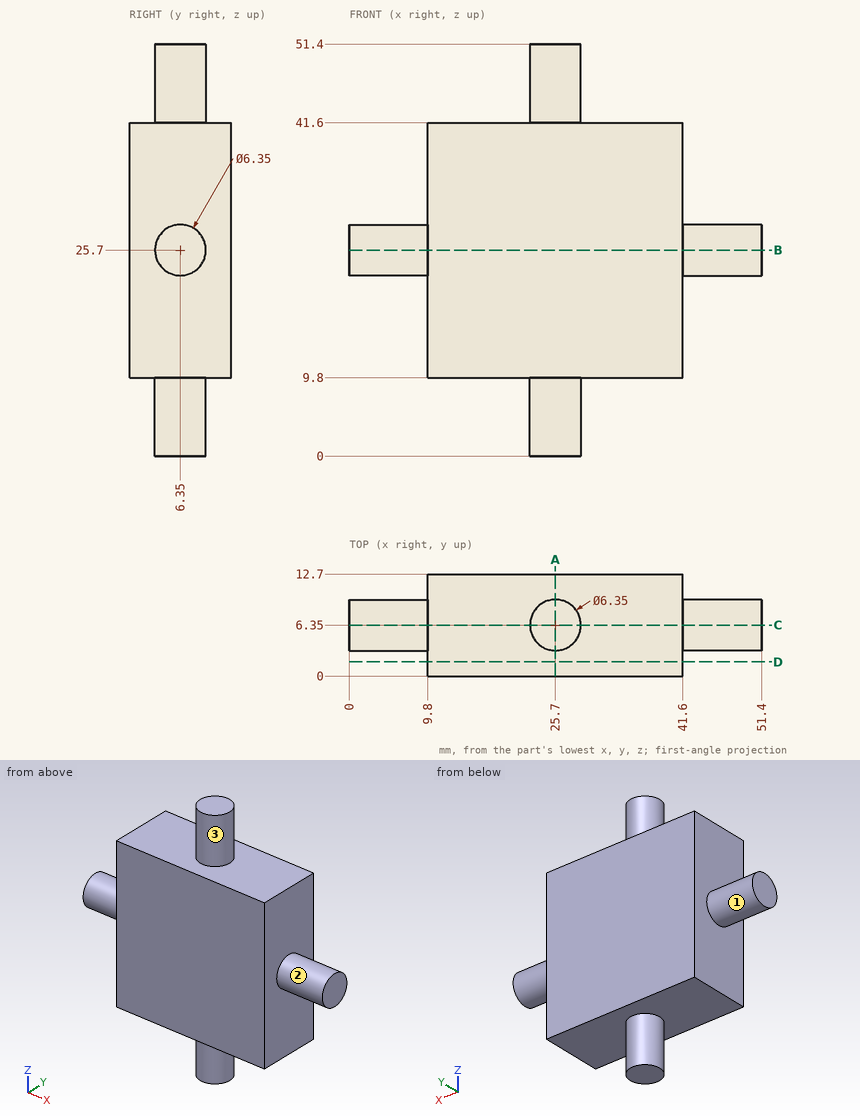
The figure shows three views and two pictorial views of one solid part (mm, origin at its lowest corner). Answer the questions. A direction names the side the tool comes from. Give positions to 0.01 mm unless a question says otherwise; leave off trailing zeros. Loops run counter-clockwise (first coordinate to the right, second up) from the corner with the lowest first, then second, coordinate; pieces in that order, holes last. Notation, with made-up numbers: (25, 34) -> (38, 34) arc R34 ccw to (38, 65) -> close; hole circle Ø6 at (59.25, -16). An arc over 180 degrees is marked (long way). Put each result on its own line as item: value. Start each with the question number.
Item 1: The part is cut by section B-B (z = 25.7). Give the vertices of the cut face in (x, y) (3 decimals), then the cut area to 3 significant figures.
Item 2: Find the intervals of material crossed by L1, parallel to X at y = 9.5, z = 20.5; L2, parallel to Y at x = 26, z = 48, in increasing order. Write a range as [from, to].
Item 3: Each of these flat-tipped pins is pushed along its axis until it touches: P1, Ø6, axis at x = 20.5, y = 2.5, coming from the -Z side; P2, Ø6, axis at x = 42.5, y = 4, coming from the +Z side; P3, Ø4, axis at y = 6, z = 20.5, coming from the +X side. Where does it stop, or does it pass through?
Item 4: The part is cut by section D-D (y = 1.75). Give the vertices of the cut face in (x, z).
Item 5: The part is cut by section A-A (x = 25.7). Give the vertices of the cut face in (y, z) (3 decimals), then the cut area to 3 significant figures.
Item 6: Which of the six approach directions +Z, -Z, +X, -X, +Y, -Y give full straight-line access (tool end or side, diameter ignored) to the marked faces 1, 2 and 3?
Item 7: The part is cut by section C-C (y = 6.35). Give the vertices of the cut face in (x, z) (3 decimals), then the cut area to 3 significant figures.
Answers below:
1. outline: (0, 3.175) -> (9.8, 3.175) -> (9.8, 0) -> (41.6, 0) -> (41.6, 3.175) -> (51.4, 3.175) -> (51.4, 9.525) -> (41.6, 9.525) -> (41.6, 12.7) -> (9.8, 12.7) -> (9.8, 9.525) -> (0, 9.525) -> close
1. area: 528 mm2
2. L1: [9.8, 41.6]
2. L2: [3.19, 9.51]
3. P1: z = 9.8
3. P2: z = 41.6
3. P3: x = 41.6
4. outline: (9.8, 9.8) -> (41.6, 9.8) -> (41.6, 41.6) -> (9.8, 41.6) -> close
5. outline: (0, 9.8) -> (3.175, 9.8) -> (3.175, 0) -> (9.525, 0) -> (9.525, 9.8) -> (12.7, 9.8) -> (12.7, 41.6) -> (9.525, 41.6) -> (9.525, 51.4) -> (3.175, 51.4) -> (3.175, 41.6) -> (0, 41.6) -> close
5. area: 528 mm2
6. face 1: -X
6. face 2: +X
6. face 3: +Z
7. outline: (0, 22.525) -> (9.8, 22.525) -> (9.8, 9.8) -> (22.525, 9.8) -> (22.525, 0) -> (28.875, 0) -> (28.875, 9.8) -> (41.6, 9.8) -> (41.6, 22.525) -> (51.4, 22.525) -> (51.4, 28.875) -> (41.6, 28.875) -> (41.6, 41.6) -> (28.875, 41.6) -> (28.875, 51.4) -> (22.525, 51.4) -> (22.525, 41.6) -> (9.8, 41.6) -> (9.8, 28.875) -> (0, 28.875) -> close
7. area: 1,260 mm2
